Geometry check sheet. Reference: the model listing, model coordinates, mm. Face numbers are marked on the shaded views. A direction names the side the tool comes from. Give positions to 0.01 mm unless a question says otherwise; leave off trailing zeros. Order: outer loops, then holes, each group sorted by start corner. A loop starts at its lowest first (then second) coordinate and runs counter-clockwise, first axis right, second up.
```python
from build123d import *

# Parameters (mm, degrees)
F0_W      = 79
F0_H      = 55
F0_W_2    = 73
F0_H_2    = 49
F1_DEPTH  = 25
F3_DEPTH  = 79
F0_W_3    = 31
F0_H_3    = 16
F4_DEPTH  = 3
F5_W      = 6
F5_H      = 4
F6_DEPTH  = 3
F5_W_2    = 37
F5_W_3    = 7
F7_DEPTH  = 6
F8_W      = 5
F8_H      = 5
F9_DEPTH  = 12.86194
F10_R     = 1.75
F11_DEPTH = 4
F12_W     = 6
F12_H     = 3
F13_DEPTH = 25
F14_DEPTH = 25


with BuildPart() as f1:
    # F0 (on Front) → F1 (new body)
    with BuildSketch(Plane.XZ):
        Rectangle(F0_W, F0_H)
        Rectangle(F0_W_2, F0_H_2, mode=Mode.SUBTRACT)
    extrude(amount=-F1_DEPTH)

    # F2 (on face) → F3 (cut, through all)
    with BuildSketch(Plane(origin=(-39.5, 0, 0), x_dir=(0, -1, 0), z_dir=(-1, 0, 0))):
        with BuildLine():
            Line((-25, -5), (-18.267742, -3.295049))
            ThreePointArc((-18.267742, -3.295049), (-12.180301, -1.187393), (-16, 4))
            Line((-16, 4), (-16.878049, 3.902439))
            Line((-16.878049, 3.902439), (-25, 3))
            Line((-25, 3), (-25, -5))
        make_face()
    extrude(amount=-F3_DEPTH, mode=Mode.SUBTRACT)

    # F0 (on Front) → F4 (join)
    with BuildSketch(Plane.XZ):
        Rectangle(F0_W_2, F0_H_2)
        with Locations((-4.921641, -1.63806)):
            Rectangle(F0_W_3, F0_H_3, mode=Mode.SUBTRACT)
    extrude(amount=-F4_DEPTH)

    # F5 (on face) → F6 (join)
    with BuildSketch(Plane(origin=(0, 3, 0), x_dir=(-1, 0, 0), z_dir=(0, 1, 0))):
        with Locations((-8.578359, -13.63806)):
            Rectangle(F5_W, F5_H)
    extrude(amount=F6_DEPTH)

    # F5 (on face) → F7 (join)
    with BuildSketch(Plane(origin=(0, 3, 0), x_dir=(-1, 0, 0), z_dir=(0, 1, 0))):
        with Locations((12.921641, -13.63806)):
            Rectangle(F5_W_2, F5_H)
        with Locations((-15.078359, -13.63806)):
            Rectangle(F5_W_3, F5_H)
    extrude(amount=F7_DEPTH)

    # F8 (on face) → F9 (join)
    with BuildSketch(Plane.XY.offset(-24.5)):
        with Locations((-6.421641, 22.5)):
            Rectangle(F8_W, F8_H)
    extrude(amount=F9_DEPTH)

    # F10 (on face) → F11 (cut, through all)
    with BuildSketch(Plane.XY.offset(-11.63806)):
        with Locations((14.828359, 5.95)):
            Circle(F10_R)
        with Locations((-28.071641, 5.95)):
            Circle(F10_R)
    extrude(amount=-F11_DEPTH, mode=Mode.SUBTRACT)

    # F12 (on face) → F13 (cut, through all)
    with BuildSketch(Plane.XZ):
        with Locations((33.5, -26)):
            Rectangle(F12_W, F12_H)
    extrude(amount=-F13_DEPTH, mode=Mode.SUBTRACT)

    # F12 (on face) → F14 (join, through all)
    with BuildSketch(Plane.XZ):
        Polygon((27.5, -27.5), (30.5, -27.5), (30.5, -24.5), (36.5, -24.5), (36.5, -21.5), (27.5, -21.5), align=None)
    extrude(amount=-F14_DEPTH)


solid = f1.part
```
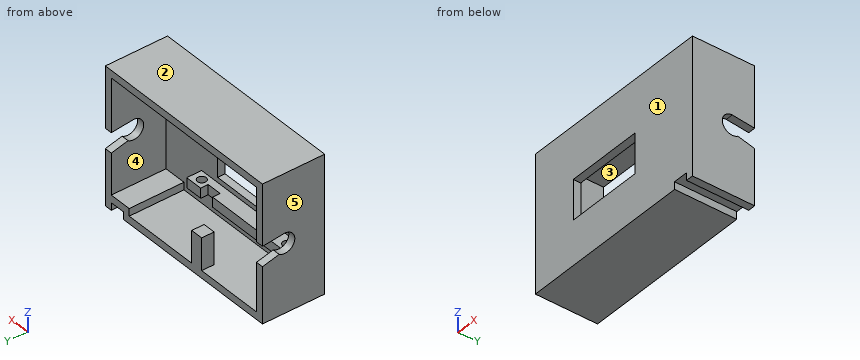
Q1. Gauge pin test, flat ends, axial feed: P1, Ø5, axis at x = -17, z = 8.5, coming from the +Y side; P2, Ø2, axis at x = 9.5, z = -13.5, coming from the +Y side; P3, Ø2, axis at x = 15.5, z = -13.5, coming from the +Y side. Record the tip position at first contact, or that the pin passes through.
Q2. Cross-section at D-D, the plane y = 10.25. Record the boundary of the cut face in (x, z).
Q3. Cross-section at B-B, the plane x = -1.5. Record the boundary of the cut face in (y, z).
Q4. Access from +Z, -Z, +X, -X, +Y, -Y to the whole of each face (thin tool, end or side, straight path). Record for the marked faces 4 and 5.
Q5. Cross-section at C-C, the plane z = 0. Record the boundary of the cut face in (x, y), and give its area (3 significant figures).
Q6. Thickness scan on L1, parallel to Z at x = 31.5, y = 12; L2, parallel to X at y = 8.25, z = -18.5; L3, parallel to Z at x = 28.5, y = 22.25. Record the ranges inside material, lowest first.
Q7. Cross-section at A-A, the plane y = 5. Record the boundary of the cut face in (x, z), and give its area (3 significant figures).
Q8. Release check for a two-part mould opening along Z. For the marked faces 1, 2 and 3 record: pulls with the +Z half, pulls with the -Z half, needs draft (parallel to the pull), parting line crosses it, or undercut.
Answers follow:
1. P1: stops at y = 3
1. P2: stops at y = 6
1. P3: stops at y = 9
2. outline: (-39.5, -27.5) - (30.5, -27.5) - (30.5, -24.5) - (36.5, -24.5) - (36.5, -27.5) - (39.5, -27.5) - (39.5, 27.5) - (-39.5, 27.5) - close; hole (-36.5, -24.5) - (27.5, -24.5) - (27.5, -21.5) - (36.5, -21.5) - (36.5, 24.5) - (-36.5, 24.5) - close
3. outline: (0, -27.5) - (25, -27.5) - (25, -24.5) - (3, -24.5) - (3, -15.64) - (9, -15.64) - (9, -11.64) - (3, -11.64) - (3, -9.64) - (0, -9.64) - close; (0, 6.36) - (3, 6.36) - (3, 24.5) - (25, 24.5) - (25, 27.5) - (0, 27.5) - close
4. face 4: +Y
4. face 5: +Z, -Z, -X, +Y, -Y
5. outline: (-39.5, 0) - (-20.42, 0) - (-20.42, 3) - (-36.5, 3) - (-36.5, 12) - (-39.5, 12) - close; (10.58, 0) - (39.5, 0) - (39.5, 12) - (36.5, 12) - (36.5, 3) - (10.58, 3) - close
5. area: 198 mm2
6. L1: z = -24.5 to -21.5, 24.5 to 27.5
6. L2: x = -39.5 to -36.5, 36.5 to 39.5
6. L3: z = -27.5 to -21.5, 24.5 to 27.5
7. outline: (-39.5, -27.5) - (30.5, -27.5) - (30.5, -24.5) - (36.5, -24.5) - (36.5, -27.5) - (39.5, -27.5) - (39.5, 27.5) - (-39.5, 27.5) - close; (-31.42, -15.64) - (-29.54, -15.64) - (-29.54, -11.64) - (-31.42, -11.64) - close; (-26.6, -15.64) - (13.36, -15.64) - (13.36, -11.64) - (-26.6, -11.64) - close; (16.3, -15.64) - (18.58, -15.64) - (18.58, -11.64) - (16.3, -11.64) - close; hole (-36.5, -24.5) - (27.5, -24.5) - (27.5, -21.5) - (36.5, -21.5) - (36.5, 24.5) - (-36.5, 24.5) - close
7. area: 953 mm2
8. face 1: needs draft
8. face 2: pulls with the +Z half
8. face 3: undercut
